Input: part model. Units: mm. Frame: model coordinates. A direction names the side the tool comes from. Coordinates: 2 decimals unless noted, no trailing zeros. Loops run counter-clockwise (first coordinate to the right, second up) from the corner with the lowest first, then second, coordinate; pieces in that order, holes last. Notation, with made-up numbers: (-24.75, 77.5) - (34.25, 77.5) arc R21 cw to (34.25, 81.5) - close; hole circle Ø6 at (86, 66.5). An arc over 180 degrees is marked (long way). Use a Markdown table: item, result. Add a question column.
1. Contact query for flat-ended pins moving along their axis: P1, Ø4.5, axis at x = 137, z = -11.5, coming from the +Y side; P2, Ø6, axis at x = 70, y = 15.5, coming from the -Z side; P3, Ø9.5, axis at x = 31.85, z = -25.4, coming from the +Y side. Output: stop coordinate, or through.
2. Section query C-C on x = 279. Return the cut outline in (y, z).
3. Draft query along Z for faces 3 (the face through (0, 6, 0)), 4 (the face through (182, 18, -4.91)), 5 (the face through (182, 18, 4.91)), 6 (the face through (332.85, 7.65, 21.91)). Return one class per face: released by +Z, released by -Z, zero draft, split by the parting line, or undercut.
4. Access query for faces 1 (the face through (333.428, 2.576, 24.385)), 2 (the face through (332.85, 7.65, -28.89)). Directions: +Z, -Z, +X, -X, +Y, -Y. A direction counts if a zero-diameter tool reaches every point of the face in a straight line with its end or side. Return the directions, or none.
5. Section query B-B on z = 25.4. Return the cut outline in (x, y), then the cut area to 3 significant figures.
6. Section query A-A on x = 336.65. Return the cut outline in (y, z).
7. Ray query, L1, parallel to Z at x = 31.85, y = 7.15; L2, parallel to X at y = 7.75, z = 25.4; L3, parallel to Z at x = 184.25, y = 3.9. Return the intervals inside material, ascending. Write a range as [from, to].
```python
from build123d import *

# Parameters (mm, degrees)
BOSS_EXTRUDE1_DEPTH                              = 368.5
CBORE_FOR_1_4_SOCKET_SHOULDER_SCREW1_D           = 6.7564
CBORE_FOR_1_4_SOCKET_SHOULDER_SCREW1_CBORE_D     = 10.31748
CBORE_FOR_1_4_SOCKET_SHOULDER_SCREW1_CBORE_DEPTH = 4.7752


with BuildPart() as part:
    # Sketch1 → Boss-Extrude1 (new body)
    with BuildSketch(Plane(origin=(0, 0, 0), x_dir=(0, 0, -1), z_dir=(1, 0, 0))):
        Polygon((-31, 0), (31, 0), (31, 10), (15.4, 10), (19.57, 15.28), (4.91, 15.28), (4.91, 21.1), (-4.91, 21.1), (-4.91, 15.28), (-19.57, 15.28), (-15.4, 10), (-31, 10), align=None)
    extrude(amount=BOSS_EXTRUDE1_DEPTH)

    # CBORE for 1/4 Socket Shoulder Screw1 (through all)
    with Locations(Plane(origin=(0, 10, 0), x_dir=(1, 0, 0), z_dir=(0, 1, 0))):
        with Locations((31.85, 25.4), (184.25, 25.4), (336.65, 25.4), (336.65, -25.4), (184.25, -25.4), (31.85, -25.4)):
            CounterBoreHole(CBORE_FOR_1_4_SOCKET_SHOULDER_SCREW1_D / 2, CBORE_FOR_1_4_SOCKET_SHOULDER_SCREW1_CBORE_D / 2, CBORE_FOR_1_4_SOCKET_SHOULDER_SCREW1_CBORE_DEPTH)


solid = part.part
```
Resolved:
| question | item | result |
|---|---|---|
| 1 | P1 | y = 15.28 |
| 1 | P2 | z = -19.57 |
| 1 | P3 | y = 5.22 |
| 2 | outline | (0, -31) - (10, -31) - (10, -15.4) - (15.28, -19.57) - (15.28, -4.91) - (21.1, -4.91) - (21.1, 4.91) - (15.28, 4.91) - (15.28, 19.57) - (10, 15.4) - (10, 31) - (0, 31) - close |
| 3 | face 3 | zero draft |
| 3 | face 4 | released by -Z |
| 3 | face 5 | released by +Z |
| 3 | face 6 | undercut |
| 4 | face 1 | +Y, -Y |
| 4 | face 2 | +Y |
| 5 | outline | (0, 0) - (28.47, 0) - (28.47, 5.22) - (26.69, 5.22) - (26.69, 10) - (0, 10) - close; (35.23, 0) - (180.87, 0) - (180.87, 5.22) - (179.09, 5.22) - (179.09, 10) - (37.01, 10) - (37.01, 5.22) - (35.23, 5.22) - close; (187.63, 0) - (333.27, 0) - (333.27, 5.22) - (331.49, 5.22) - (331.49, 10) - (189.41, 10) - (189.41, 5.22) - (187.63, 5.22) - close; (340.03, 0) - (368.5, 0) - (368.5, 10) - (341.81, 10) - (341.81, 5.22) - (340.03, 5.22) - close |
| 5 | area | 3,430 mm² |
| 6 | outline | (0, -31) - (10, -31) - (10, -30.56) - (5.22, -30.56) - (5.22, -28.78) - (0, -28.78) - close; (0, -22.02) - (5.22, -22.02) - (5.22, -20.24) - (10, -20.24) - (10, -15.4) - (15.28, -19.57) - (15.28, -4.91) - (21.1, -4.91) - (21.1, 4.91) - (15.28, 4.91) - (15.28, 19.57) - (10, 15.4) - (10, 20.24) - (5.22, 20.24) - (5.22, 22.02) - (0, 22.02) - close; (0, 28.78) - (5.22, 28.78) - (5.22, 30.56) - (10, 30.56) - (10, 31) - (0, 31) - close |
| 7 | L1 | [-31, -30.56], [-20.24, 20.24], [30.56, 31] |
| 7 | L2 | [0, 26.69], [37.01, 179.09], [189.41, 331.49], [341.81, 368.5] |
| 7 | L3 | [-31, -28.78], [-22.02, 22.02], [28.78, 31] |
